Verification items for the finished model (mm, model axes). A direction names the side the tool comes from. Give positions to 0.01 mm unless a question says otherwise; leave off trailing zeros. Write each loop counter-clockwise with the first axis right and the second up, starting at its lowest first coordinate (ties: lowest second). Pieces come first, ordered by that corner, then holes. Notation, with made-up numbers: (-39.75, 29.25) -> (10.25, 29.25) arc R5 cw to (10.25, 34.25) -> close; hole circle Ø3 at (37.5, 68.5). An arc over 180 degrees is marked (long way). Write item = value, one per line.
from build123d import *

# Parameters (mm, degrees)
SKETCH1_R               = 7.5
BOSS_EXTRUDE1_DEPTH     = 20
SKETCH4_R               = 7.5
SKETCH4_R_2             = 6
CUT_EXTRUDE2_DEPTH      = 2.5
CUT_EXTRUDE2_DEPTH_BACK = 2.5


with BuildPart() as part:
    # Sketch1 → Boss-Extrude1 (new body)
    with BuildSketch(Plane.XY):
        Circle(SKETCH1_R)
    extrude(amount=-BOSS_EXTRUDE1_DEPTH)

    # Sketch4 → Cut-Extrude2 (cut, two sides)
    with BuildSketch(Plane.XY.offset(-7.5)) as cut_extrude2_sk:
        Circle(SKETCH4_R)
        Circle(SKETCH4_R_2, mode=Mode.SUBTRACT)
    extrude(amount=CUT_EXTRUDE2_DEPTH, mode=Mode.SUBTRACT)
    extrude(cut_extrude2_sk.sketch, amount=-CUT_EXTRUDE2_DEPTH_BACK, mode=Mode.SUBTRACT)


solid = part.part
Item 1: Mould release check, pull along Z, two halves, no side actions. Record for faces 1 (the flat face through (0, 0, 0)), 2 (the flat face through (2, 6, -5)), 3 (the cylindrical face through (-7.493, 0.33, -2.465)): +Z half, -Z half, draft (parallel to the pull), parting line (faces both ways), or undercut.
Response values:
face_1 = +Z half
face_2 = undercut
face_3 = draft
Item 2: Sectioned sample at B-B on y = 0. Record the cut outline in (x, z), then the cut area to 3 significant figures.
Response values:
outline = (-7.5, -20) -> (7.5, -20) -> (7.5, -10) -> (6, -10) -> (6, -5) -> (7.5, -5) -> (7.5, 0) -> (-7.5, 0) -> (-7.5, -5) -> (-6, -5) -> (-6, -10) -> (-7.5, -10) -> close
area = 285 mm^2
Item 3: Material ranges on line 1 (Z direction, x = -3.5, y = 6.25); line 2 (Y direction, x = 4.25, z = -2.75); line 3 (X direction, y = 1.75, z = -13.75), recorded low to high.
Response values:
line_1 = -20 to -10, -5 to 0
line_2 = -6.18 to 6.18
line_3 = -7.29 to 7.29
Item 4: Go/stop test with flat-tipped pins: P1, Ø1, axis at x = 5, z = -15, coming from the -Y side; P2, Ø1.5, axis at x = 4.5, z = -16.5, coming from the -Y side; P3, Ø6, axis at y = -4, z = -17, coming from the -X side; P4, Ø2, axis at x = 3.5, y = -5, coming from the +Z side. Record where each tip stops, or that it passes through.
Response values:
P1 = -6
P2 = -6.5
P3 = -7.43
P4 = 0
Item 5: Sectioned sample at A-A on x = 6.5. Record the cut outline in (y, z), then the cut area to 3 significant figures.
Response values:
outline = (-3.74, -20) -> (3.74, -20) -> (3.74, -10) -> (-3.74, -10) -> close; (-3.74, -5) -> (3.74, -5) -> (3.74, 0) -> (-3.74, 0) -> close
area = 112 mm^2
Item 6: Sectioned sample at D-D on z = -14. Record the cut outline in (x, y).
Response values:
outline = circle Ø15 at (0, 0)
Item 7: Set-up check for faces 4 (the flat face through (2, 6, -10)), 5 (the cylindrical face through (-7.493, 0.33, -14.93)): record each of +Z, -Z, +X, -X, +Y, -Y from which the full face is reachable in a straight line by a thin tool's end or side.
Response values:
face_4 = none
face_5 = +Z, -Z
